```python
from build123d import *

# Parameters (mm, degrees)
SKETCH_1_R      = 2.2
SKETCH_1_R_2    = 1.7
EXTRUDE_1_DEPTH = 5


with BuildPart() as part:
    # 草图1 → 凸台-拉伸1 (new body)
    with BuildSketch(Plane(origin=(0, 0, 0), x_dir=(1, 0, 0), z_dir=(0, 1, 0))):
        with BuildLine():
            Line((0, 5), (34.118365096, 5))
            Line((34.118365096, 5), (42.686825491, 8.118664537))
            ThreePointArc((42.686825491, 8.118664537), (49.095389312, 5.13030215), (46.107026924, -1.278261671))
            Line((46.107026924, -1.278261671), (37.53856653, -4.396926208))
            ThreePointArc((37.53856653, -4.396926208), (35.854846873, -4.84807753), (34.118365096, -5))
            Line((34.118365096, -5), (0, -5))
            ThreePointArc((0, -5), (-5, 0), (0, 5))
        make_face()
        with Locations(Location((0, 0, 0), (0, 0, 270))):
            Circle(SKETCH_1_R, mode=Mode.SUBTRACT)
        with Locations(Location((20, 0, 0), (0, 0, 270))):
            Circle(SKETCH_1_R, mode=Mode.SUBTRACT)
        with Locations(Location((35, 0, 0), (0, 0, 270))):
            Circle(SKETCH_1_R_2, mode=Mode.SUBTRACT)
        with Locations(Location((44.396926208, 3.420201433, 0), (0, 0, 270))):
            Circle(SKETCH_1_R_2, mode=Mode.SUBTRACT)
    extrude(amount=EXTRUDE_1_DEPTH)


solid = part.part
```
Input: part model. Units: mm. Frame: model coordinates. A direction names the side the tool comes from. Give positions to 0.01 mm unless a question says otherwise; leave off trailing zeros. Order: outer loops, then holes, each group sorted by start corner. A loop starts at its lowest first (then second) coordinate and runs counter-clockwise, first axis right, second up. Notation, with made-up numbers: M 87.25,57.25 L 110.25,57.25 A24 cw 110.25,85.25 Z; hole C 84.5,25.5 d8. An arc over 180 degrees is marked long. Return JSON: item names as keys, results as strings.
Item 1: Pull-direction query (X, two-part tool) for faces 3 (the cylindrical face through (17.852, 2.465, -0.477)), 4 (the flat face through (41.883, 2.465, 2.816)), 5 (the cylindrical face through (33.34, 2.46, -0.37)), 6 (the cylindrical face through (-5, 2, 0)); classes: +X half, -X half, draft (parallel to the pull), parting line (faces both ways), or undercut.
Solutions:
{"face 3": "undercut", "face 4": "+X half", "face 5": "undercut", "face 6": "-X half"}
Item 2: Cut plane A-A (x = 20). Return loops of the section in (y, z).
Solutions:
{"outline": "M 0,-5 L 5,-5 L 5,-2.2 L 0,-2.2 Z; M 0,2.2 L 5,2.2 L 5,5 L 0,5 Z"}
Item 3: Cut plane D-D (y = 3.85). Return loops of the section in (x, z).
Solutions:
{"outline": "M 0,-5 L 34.12,-5 L 42.69,-8.12 A5 ccw 46.11,1.28 L 37.54,4.4 A10 ccw 34.12,5 L 0,5 A5 ccw Z; hole C 0,0 d4.4; hole C 20,0 d4.4; hole C 35,0 d3.4; hole C 44.4,-3.42 d3.4"}
Item 4: Access query for faces 1 (the flat face through (17, 2, -5)), 2 (the flat face through (23, 0, 0)). Directions: +Z, -Z, +X, -X, +Y, -Y. A direction counts if a zero-diameter tool reaches every point of the face in a straight line with its end or side. Return the directions, or none.
Solutions:
{"face 1": "-Z, -X, +Y, -Y", "face 2": "+Z, -Z, +X, -X, -Y"}
Item 5: First-contact query: P1, Ø2.5, axis at x = 35, z = 0, coming from the +Y side; P2, Ø3, axis at x = 4, y = 2, coming from the -Z side; P3, Ø2, axis at y = 3, z = 0, coming from the +X side; P4, Ø2, axis at y = 3.5, z = -1.5, coming from the -X side. Flat tips, straight axial feed; report the tip coordinate or a pass-through.
Solutions:
{"P1": "through", "P2": "z = -5", "P3": "x = 48.77", "P4": "x = -4.97"}
Item 6: Cut plane C-C (z = -2.75). Return loops of the section in (x, y), then the cut area to 3 significant figures.
Solutions:
{"outline": "M -4.18,0 L 42.83,0 L 42.83,5 L -4.18,5 Z; M 45.96,0 L 49.35,0 L 49.35,5 L 45.96,5 Z", "area": "252 mm^2"}
Item 7: Ray query, probe 1 along X at (y, z) = (2.35, 0); probe 2 along X at (y, z) = (2, -1.5); probe 3 along Z at (x, y) = (5, 3.1). Return the intervals inside material, ascending.
Solutions:
{"probe 1": "-5 to -2.2, 2.2 to 17.8, 22.2 to 33.3, 36.7 to 48.04", "probe 2": "-4.77 to -1.61, 1.61 to 18.39, 21.61 to 34.2, 35.8 to 49.01", "probe 3": "-5 to 5"}
Item 8: Cut plane B-B (z = 0.5). Return loops of the section in (x, y).
Solutions:
{"outline": "M -4.97,0 L -2.14,0 L -2.14,5 L -4.97,5 Z; M 2.14,0 L 17.86,0 L 17.86,5 L 2.14,5 Z; M 22.14,0 L 33.38,0 L 33.38,5 L 22.14,5 Z; M 36.62,0 L 47.5,0 L 47.5,5 L 36.62,5 Z"}
